from build123d import *

# Parameters (mm, degrees)
F_90_0_0087_DIAMETER_HOLE1_D = 0.22098
CIRPATTERN3_COUNT            = 3
SKETCH8_R                    = 80.01
SKETCH8_R_2                  = 55.626
CUT_EXTRUDE1_DEPTH           = 10
FILLET5_R                    = 4
CHAMFER1_SIZE                = 4
SKETCH10_R                   = 84.55
SKETCH10_R_2                 = 82.55
BOSS_EXTRUDE1_DEPTH          = 7.5
CHAMFER3_SIZE                = 5
CHAMFER3_SIZE2               = 8.660254038
FILLET4_R                    = 5
F_12_0_189_DIAMETER_HOLE1_D  = 4.8006
CIRPATTERN5_COUNT            = 3


with BuildPart() as part:
    # Sketch2 → Revolve1 (revolve)
    with BuildSketch(Plane(origin=(0, 0, 0), x_dir=(0, 0, -1), z_dir=(1, 0, 0))):
        Polygon((-45.8, 0), (-82.55, 0), (-82.55, 12.7), (-50.8, 12.7), (-50.8, 5.2), (-45.8, 5.2), align=None)
    revolve(axis=Axis((0, -0.635, 0), (0, 1, 0)))

    # #90 (0.0087) Diameter Hole1 (through all)
    with Locations(Plane(origin=(0, 12.7, 0), x_dir=(1, 0, 0), z_dir=(0, 1, 0))):
        with Locations((-35, 60.621778265)):
            f_90_0_0087_diameter_hole1 = Hole(F_90_0_0087_DIAMETER_HOLE1_D / 2)

    # CirPattern3: #90 (0.0087) Diameter Hole1 ×3 about axis
    cirpattern3_axis = Axis((0, 0, 0), (0, 1, 0))
    for i in range(1, CIRPATTERN3_COUNT):
        add(f_90_0_0087_diameter_hole1.rotate(cirpattern3_axis, i * 360 / CIRPATTERN3_COUNT), mode=Mode.SUBTRACT)

    # Sketch8 → Cut-Extrude1 (cut)
    with BuildSketch(Plane(origin=(0, 12.7, 0), x_dir=(1, 0, 0), z_dir=(0, 1, 0))):
        Circle(SKETCH8_R)
        Circle(SKETCH8_R_2, mode=Mode.SUBTRACT)
    extrude(amount=-CUT_EXTRUDE1_DEPTH, mode=Mode.SUBTRACT)

    # Fillet5
    fillet5_edges = [part.edges().sort_by_distance(p)[0] for p in [
        (-55.626, 2.7, 0),
        (-80.01, 2.7, 0),
    ]]
    fillet(fillet5_edges, radius=FILLET5_R)

    # Chamfer1
    chamfer1_edges = [part.edges().sort_by_distance(p)[0] for p in [
        (0, 0, -45.8),
    ]]
    chamfer(chamfer1_edges, length=CHAMFER1_SIZE)

    # Sketch10 → Boss-Extrude1 (add)
    with BuildSketch(Plane.XZ):
        Circle(SKETCH10_R)
        Circle(SKETCH10_R_2, mode=Mode.SUBTRACT)
    extrude(amount=-BOSS_EXTRUDE1_DEPTH)

    # Chamfer3
    chamfer3_edges = [part.edges().sort_by_distance(p)[0] for p in [
        (-84.55, 0, 0),
    ]]
    chamfer3_side = [part.faces().sort_by_distance(p)[0] for p in [
        (-84.55, 3.75, 0),
    ]]
    chamfer(chamfer3_edges, length=CHAMFER3_SIZE, length2=CHAMFER3_SIZE2, reference=chamfer3_side[0])

    # Fillet4
    fillet4_edges = [part.edges().sort_by_distance(p)[0] for p in [
        (-75.889745962, 0, 0),
    ]]
    fillet(fillet4_edges, radius=FILLET4_R)

    # #12 (0.189) Diameter Hole1 (through all)
    with Locations(Plane(origin=(0, 0, 0), x_dir=(-1, 0, 0), z_dir=(0, -1, 0))):
        with Locations((35, 60.621778265)):
            f_12_0_189_diameter_hole1 = Hole(F_12_0_189_DIAMETER_HOLE1_D / 2)

    # CirPattern5: #12 (0.189) Diameter Hole1 ×3 about axis
    cirpattern5_axis = Axis((0, 0, 0), (0, 1, 0))
    for i in range(1, CIRPATTERN5_COUNT):
        add(f_12_0_189_diameter_hole1.rotate(cirpattern5_axis, i * 360 / CIRPATTERN5_COUNT), mode=Mode.SUBTRACT)


solid = part.part
Here's how the part is built. I have some questions about the finished solid (model axes, mm). A direction names the side the tool comes from. Round coordinates to 2 decimals unless told otherwise and drop trailing zeros. Use CSV: the item, a comma, the result in double quotes.
1. I'm going to push flat-ended pins straight in: P1, Ø5, axis at y = 9.5, z = -46, coming from the +X side; P2, Ø4, axis at x = 64.5, z = -14.5, coming from the +Y side; P3, Ø2, axis at x = -46, y = 5, coming from the +Z side; P4, Ø4.5, axis at x = -35, z = 60.62, coming from the -Y side. Where does each tip first touch, or does it pass through?
Recorded:
P1,"stops at x = 71.89"
P2,"stops at y = 2.7"
P3,"stops at z = 71.58"
P4,"passes through"
2. Which directions (+Z, -Z, +X, -X, +Y, -Y) give clear straight access to the entire face, cutting with the end or side of a thin tool? Please do faces 4 (the face through (49, 0, -16)), 5 (the face through (45.4, 5.2, -7.8)).
Recorded:
face 4,"+Z, -Z, +X, -X, -Y"
face 5,"+Y"
3. I need wall thicknesses on line 1 along X through (y, z) = (11, 0); line 2 along X through (y, z) = (6, 5.5); line 3 along X through (y, z) = (8, 51). Which ranges of each line are inside material? Lowest first, please.
Recorded:
line 1,"x = -82.55 to -80.01, -55.63 to -50.8, 50.8 to 55.63, 80.01 to 82.55"
line 2,"x = -84.37 to -79.76, -55.42 to -50.5, 50.5 to 55.42, 79.76 to 84.37"
line 3,"x = -64.91 to -61.65, -22.21 to 22.21, 61.65 to 64.91"
4. Thinking about a two-plate mould opening in Z: for faces 1 (the face through (43, 12.7, -68)), 2 (the face through (-10.078, 0.88, 76.755)), 3 (the face through (76.315, 9.742, -24.033)), which applies, pulls with the +Z half, pulls with the -Z half, needs draft (parallel to the pull), parting line crosses it, or undercut?
Recorded:
face 1,"needs draft"
face 2,"parting line crosses it"
face 3,"undercut"
5. I want a section at B-B on z = 0. Give the number of separate pieces and of enclosed holes in the cut face, and give its area (3 significant figures).
Recorded:
separate pieces,"3"
enclosed holes,"0"
area,"342 mm2"
